Work out the finished part from the listing and answer in its coordinate system (mm). Face numbers are marked on the shaded views. A direction names the side the tool comes from. Round coordinates to 2 decimals unless told otherwise and drop trailing zeros. Order: outer loops, then holes, each group sorted by start corner. A loop starts at its lowest first (then second) coordinate and runs counter-clockwise, first axis right, second up. Notation, with made-up numbers: (75, 11) -> (111, 11) arc R23 ccw to (111, 40) -> close; hole circle Ø6 at (52, 71.5). An arc over 180 degrees is marked (long way). Use one line per item in the form item = value.
Autodesk Inventor part; units mm, degrees
ref_plane "YZ Plane" through (0, 0, 0) normal (1, 0, 0) x (0, 1, 0)
ref_plane "XZ Plane" through (0, 0, 0) normal (0, 1, 0) x (-1, 0, 0)
ref_plane "XY Plane" through (0, 0, 0) normal (0, 0, 1) x (1, 0, 0)
sketch "Sketch1" plane through (0, 0, 0) normal (0, 1, 0) x (-1, 0, 0)
  line L0 (-36, -36) -> (0, -36)
  line L1 (0, -36) -> (0, 0)
  line L2 (-11.2353, -15.6026) -> (-15.4779, -11.36)
  line L3 (-15.4779, -7.1174) -> (-6.3606, 2)
  line L4 (2, -6.61) -> (-6.9926, -15.6026)
  circle A0 centre (-25.4718, -10.6529) radius 1.5
  line L5 (-15.4779, -7.1174) -> (-15.4779, -11.36)
  line L6 (-6.9926, -15.6026) -> (-11.2353, -15.6026)
  line L7 (-20.5221, -7.1174) -> (-29.6394, 2)
  line L8 (-38, -6.61) -> (-29.0074, -15.6026)
  line L9 (-24.7647, -15.6026) -> (-20.5221, -11.36)
  line L10 (-20.5221, -7.1174) -> (-20.5221, -11.36)
  line L11 (-29.0074, -15.6026) -> (-24.7647, -15.6026)
  line L12 (-15.4779, -28.8826) -> (-6.3606, -38)
  line L13 (2, -29.39) -> (-6.9926, -20.3974)
  line L14 (-11.2353, -20.3974) -> (-15.4779, -24.64)
  line L15 (-15.4779, -28.8826) -> (-15.4779, -24.64)
  line L16 (-6.9926, -20.3974) -> (-11.2353, -20.3974)
  line L17 (-20.5221, -28.8826) -> (-20.5221, -24.64)
  line L18 (-24.7647, -20.3974) -> (-20.5221, -24.64)
  line L19 (-20.5221, -28.8826) -> (-29.6394, -38)
  line L20 (-29.0074, -20.3974) -> (-24.7647, -20.3974)
  line L21 (-38, -29.39) -> (-29.0074, -20.3974)
  line L22 (0, 0) -> (-36, 0)
  line L23 (-36, 0) -> (-36, -36)
  circle A1 centre (-10.5282, -25.3471) radius 1.5
  circle A2 centre (-25.4718, -25.3471) radius 1.5
  circle A3 centre (-10.5282, -10.6529) radius 1.5
  line L24 (2, -38) -> (2, 2)
  line L25 (2, 2) -> (-38, 2)
  line L26 (-38, 2) -> (-38, -38)
  line L27 (-38, -38) -> (2, -38)
  circle A4 centre (-2.75, -2.75) radius 1.5
  circle A5 centre (-33.25, -2.75) radius 1.5
  circle A6 centre (-33.25, -33.25) radius 1.5
  circle A7 centre (-2.75, -33.25) radius 1.5
  point P0 (-9.114, -18.276)
  point P1 (-17.5992, -26.7613)
  point P2 (-26.886, -18.276)
  point P3 (-18.4008, -26.7613)
  point P4 (-9.114, -17.724)
  point P5 (-17.5992, -9.2387)
  point P6 (-18.4008, -9.2387)
  point P7 (-26.886, -17.724)
  dimension "d0" = 36
  dimension "d55" = 36
  dimension "d56" = 40
  dimension "d57" = 40
  dimension "d58" = 3
  dimension "d59" = 3
  dimension "d60" = 3
  dimension "d61" = 3
extrude "Extrusion5" add sketch "Sketch1" along normal blind 3
extrude "Extrusion6" add sketch "Sketch1" along normal blind 7 contours L19 L17 L18 L20 L21 L23 L8 L11 L9 L10 L7 L22 L3 L5 L2 L6 L4 L1 L13 L16 L14 L15 L12 L0 | L0 L12 L27 L19 | L21 L26 L8 L23 | L1 L4 L24 L13 | L7 L25 L3 L22
fillet "Fillet2" radius 2 4 edges at (38, 1.5, 2) (-2, 1.5, 2) (-2, 1.5, -38) (38, 1.5, -38)
sketch "Sketch2" plane through (0, 7, 0) normal (0, 1, 0) x (1, 0, 0)
  circle A0 centre (1, 18) radius 1.5
  circle A1 centre (18, 35) radius 1.5
  circle A2 centre (35, 18) radius 1.5
  point P0 (0, 0)
  dimension "d56" = 40
  dimension "d68" = 3
  dimension "d71" = 3
  dimension "d72" = 3
properties part number "Bot"
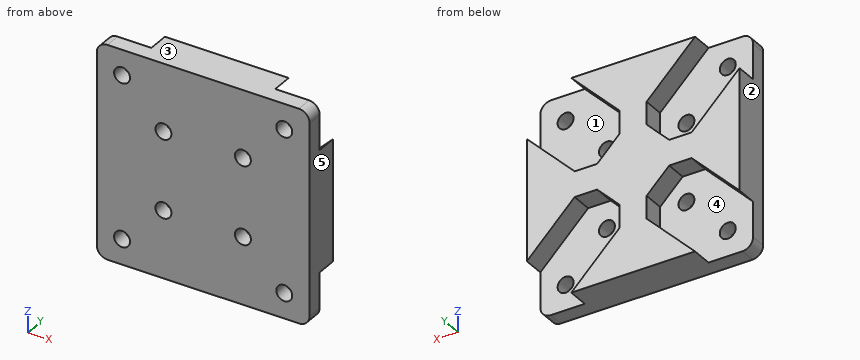
Item 1: Flat-ended cylindrical pins translate along their axes: P1, Ø3.5, axis at x = 33.25, z = -2.75, coming from the +Y side; P2, Ø3.5, axis at x = 2.75, z = -2.75, coming from the -Y side. Find the tip coordinate at first contact, or state that the pin passes through.
Findings:
P1 = 3
P2 = 0
Item 2: The part is cut by section A-A, the plane x = 2.75. Give the vertices of the cut face in (y, z).
Findings:
outline = (0, -38) -> (3, -38) -> (3, -34.75) -> (0, -34.75) -> close; (0, -31.75) -> (3, -31.75) -> (3, -24.64) -> (7, -24.64) -> (7, -11.36) -> (3, -11.36) -> (3, -4.25) -> (0, -4.25) -> close; (0, -1.25) -> (3, -1.25) -> (3, 2) -> (0, 2) -> close
Item 3: The part is cut by section D-D, the plane z = -28. Give the vertices of the cut face in (x, y).
Findings:
outline = (-2, 0) -> (38, 0) -> (38, 7) -> (36.61, 7) -> (36.61, 3) -> (20.52, 3) -> (20.52, 7) -> (15.48, 7) -> (15.48, 3) -> (-0.61, 3) -> (-0.61, 7) -> (-2, 7) -> close
Item 4: The part is cut by section B-B, the plane z = -2.75. Give the vertices of the cut face in (x, y).
Findings:
outline = (-2, 0) -> (1.25, 0) -> (1.25, 3) -> (-2, 3) -> close; (4.25, 0) -> (31.75, 0) -> (31.75, 3) -> (24.89, 3) -> (24.89, 7) -> (11.11, 7) -> (11.11, 3) -> (4.25, 3) -> close; (34.75, 0) -> (38, 0) -> (38, 3) -> (34.75, 3) -> close
Item 5: For the marked faces 1 and 2, determine the directions among +Z, -Z, +X, -X, +Y, -Y from which every point of the face is accessible in a straight line to the end or side of a thin tool.
Findings:
face_1 = +Y
face_2 = +Z, -Z, -X, +Y, -Y
Item 6: Consider line 1 along Z through (x, y) = (2.75, 1.7); line 2 along Z through (x, y) = (11, 6.25); line 3 along X through (y, z) = (1, -1.5). Determine where each line is inside the solid, lowest interval first.
Findings:
line_1 = -38 to -34.75, -31.75 to -4.25, -1.25 to 2
line_2 = -38 to -33.36, -20.4 to -15.6, -2.64 to 2
line_3 = -2 to 1.92, 3.58 to 32.42, 34.08 to 38
Item 7: Determine the mould class of the marked faces 3, 4 and 5 for opening direction X: released by +X, released by -X, zero draft, split by the parting line, or undercut.
Findings:
face_3 = zero draft
face_4 = undercut
face_5 = released by +X
Item 8: The part is cut by section C-C, the plane y = 5. Give the vertices of the cut face in (x, z), and give its area (3 significant figures).
Findings:
outline = (-2, -29.39) -> (6.99, -20.4) -> (11.24, -20.4) -> (15.48, -24.64) -> (15.48, -28.88) -> (6.36, -38) -> (29.64, -38) -> (20.52, -28.88) -> (20.52, -24.64) -> (24.76, -20.4) -> (29.01, -20.4) -> (38, -29.39) -> (38, -6.61) -> (29.01, -15.6) -> (24.76, -15.6) -> (20.52, -11.36) -> (20.52, -7.12) -> (29.64, 2) -> (6.36, 2) -> (15.48, -7.12) -> (15.48, -11.36) -> (11.24, -15.6) -> (6.99, -15.6) -> (-2, -6.61) -> close
area = 733 mm^2
